from build123d import *

# Parameters (mm, degrees)
MODEL_R                 = 1.5
SALIENTE_EXTRUIR1_DEPTH = 3


with BuildPart() as part:
    # Model → Saliente-Extruir1 (new body)
    with BuildSketch(Plane.XY):
        with BuildLine():
            Line((185.972853309, 282.646547335), (178.597853309, 282.646547335))
            Line((178.597853309, 282.646547335), (178.597853309, 264.646547335))
            Line((178.597853309, 264.646547335), (201.097853309, 264.646547335))
            ThreePointArc((201.097853309, 264.646547335), (205.597853309, 269.146547335), (201.097853309, 273.646547335))
            Line((201.097853309, 273.646547335), (189.222853309, 273.646547335))
            ThreePointArc((189.222853309, 273.646547335), (188.07380479, 274.122498816), (187.597853309, 275.271547335))
            Line((187.597853309, 275.271547335), (187.597853309, 281.021547335))
            ThreePointArc((187.597853309, 281.021547335), (187.121901829, 282.170595855), (185.972853309, 282.646547335))
        make_face()
        with Locations((201.097853309, 269.146547335)):
            Circle(MODEL_R, mode=Mode.SUBTRACT)
        with Locations((183.097853309, 278.145968764)):
            Circle(MODEL_R, mode=Mode.SUBTRACT)
        with BuildLine():
            Line((182.222853309, 265.896547335), (183.972853309, 265.896547335))
            ThreePointArc((183.972853309, 265.896547335), (184.503183395, 266.116217249), (184.722853309, 266.646547335))
            Line((184.722853309, 266.646547335), (184.722853309, 271.646547335))
            ThreePointArc((184.722853309, 271.646547335), (184.503183395, 272.176877421), (183.972853309, 272.396547335))
            Line((183.972853309, 272.396547335), (182.222853309, 272.396547335))
            ThreePointArc((182.222853309, 272.396547335), (181.692523223, 272.176877421), (181.472853309, 271.646547335))
            Line((181.472853309, 271.646547335), (181.472853309, 266.646547335))
            ThreePointArc((181.472853309, 266.646547335), (181.692523223, 266.116217249), (182.222853309, 265.896547335))
        make_face(mode=Mode.SUBTRACT)
    extrude(amount=SALIENTE_EXTRUIR1_DEPTH)


solid = part.part
The model under review builds one solid part; all positions refer to its coordinate system, in mm. A direction names the side the tool comes from. Give positions to 0.01 mm unless a question says otherwise; leave off trailing zeros. Write each loop counter-clockwise with the first axis right and the second up, starting at its lowest first coordinate (ties: lowest second). Pieces come first, ordered by that corner, then holes.
1. Add section A-A, the plane y = 278.5. Write out the cut boundary in (x, z).
2. For P1, Ø1.5, axis at y = 271, z = 0.5, coming from the +X side; P2, Ø1.5, axis at x = 199, z = 2, coming from the +Y side, all flat-tipped, find the tip position at first contact; note any pin that passes through.
3. Add section C-C, the plane z = 1.7. Write out the cut boundary in (x, y) (3 decimals), plus the area to 3 significant figures.
4. Add section D-D, the plane y = 276. Write out the cut boundary in (x, z).
5. Wall thickness on L1, parallel to Y at x = 184, z = 0.3; L2, parallel to X at y = 270.5, z = 1.6; L3, parallel to Y at x = 195.75, z = 1: over which ranges is each line inside the solid? List them lowest first.
6. Add section B-B, the plane x = 201.5. Write out the cut boundary in (y, z).
7. Tool access review of faces 4 (the flat face through (187.598, 278, 1)), 5 (the flat face through (189, 272, 0)), 6 (the flat face through (183, 265.897, 1)): name each direction out of +Z, -Z, +X, -X, +Y, -Y from which nothing blocks a thin tool from reaching the whole face with its end or side.
8. Draft analysis for pull direction Y (two halves, no side actions). For faces 1 (the flat face through (182, 282.647, 1)), 2 (the flat face through (178.598, 274, 1)), 3 (the cylindrical face through (181.6, 278.2, 1.5)), state which applies: +Y half, -Y half, draft (parallel to the pull), parting line (faces both ways), or undercut.
Worked answers:
1. outline: (178.6, 0) - (181.64, 0) - (181.64, 3) - (178.6, 3) - close; (184.56, 0) - (187.6, 0) - (187.6, 3) - (184.56, 3) - close
2. P1: stops at x = 205.46
2. P2: stops at y = 273.65
3. outline: (178.598, 264.647) - (201.098, 264.647) arc R4.5 ccw to (201.098, 273.647) - (189.223, 273.647) arc R1.625 cw to (187.598, 275.272) - (187.598, 281.022) arc R1.625 ccw to (185.973, 282.647) - (178.598, 282.647) - close; hole (181.473, 266.647) arc R0.75 ccw to (182.223, 265.897) - (183.973, 265.897) arc R0.75 ccw to (184.723, 266.647) - (184.723, 271.647) arc R0.75 ccw to (183.973, 272.397) - (182.223, 272.397) arc R0.75 ccw to (181.473, 271.647) - close; hole circle Ø3 at (183.098, 278.146); hole circle Ø3 at (201.098, 269.147)
3. area: 281 mm2
4. outline: (178.6, 0) - (187.6, 0) - (187.6, 3) - (178.6, 3) - close
5. L1: y = 264.65 to 265.9, 272.4 to 276.95, 279.34 to 282.65
5. L2: x = 178.6 to 181.47, 184.72 to 200.45, 201.74 to 205.39
5. L3: y = 264.65 to 273.65
6. outline: (264.66, 0) - (267.7, 0) - (267.7, 3) - (264.66, 3) - close; (270.59, 0) - (273.63, 0) - (273.63, 3) - (270.59, 3) - close
7. face 4: +Z, -Z, +X, +Y
7. face 5: -Z, +X, -X, +Y, -Y
7. face 6: +Z, -Z
8. face 1: +Y half
8. face 2: draft
8. face 3: undercut
